Source: CAD feature listing. Evaluate the final solid. Frame: model axes, mm. A direction names the side the tool comes from. Give positions to 0.01 mm unless a question says otherwise; leave off trailing zeros. Order: outer loops, then holes, each group sorted by start corner. A loop starts at its lowest first (then second) coordinate and runs counter-clockwise, first axis right, second up.
1) Section C-C, the plane z = -31. Return loops of the section in (x, y).
2) Draft query along X for faces 3 (the face through (-50.503, 3.042, -109.333)), 4 (the face through (-2, 3, 138)). Return one class per face: released by +X, released by -X, zero draft, split by the parting line, or undercut.
3) Material intervals for line 1 (X direction, y = 2.4, z = 55); line 2 (Z direction, x = 128, y = 4.35); line 3 (X direction, y = 2.6, z = -60), sorted ascending.
4) Section A-A, the plane x = -66.5. Return loops of the section in (y, z), plus the area to 3 significant figures.
5) Section B-B, the plane z = 35.5. Return loops of the section in (x, y), plus the area to 3 significant figures.
6) Access query for faces 1 (the face through (2.377, 3.042, -33.695)), 2 (the face through (-2, 3, -138)). Directions: +Z, -Z, +X, -X, +Y, -Y. A direction counts if a zero-diameter tool reaches every point of the face in a straight line with its end or side. Return the directions, or none.
7) Section D-D, the plane y = 1.35. Give the number of separate pieces and of enclosed holes in the cut face, plus the area to 3 significant figures.
```python
from build123d import *

# Parameters (mm, degrees)
SKETCH_1_W                = 276
SKETCH_1_H                = 276
EXTRUDE_1_DEPTH           = 6
FILLET_1_R                = 2
SKETCH_2_R                = 2
CUT_EXTRUDE_1_DEPTH       = 6
SKETCH_3_R                = 2
CUT_EXTRUDE_150_164_DEPTH = 6
SKETCH_4_R                = 2
CUT_EXTRUDE_94_94_DEPTH   = 6
SKETCH_7_R                = 1.75
JETSON_DEPTH              = 6
SKETCH_8_R                = 1.75
CUT_EXTRUDE_7_DEPTH       = 6
SKETCH_9_R                = 1.8
CUT_EXTRUDE_8_DEPTH       = 6
CUT_EXTRUDE_5_DEPTH       = 6


with BuildPart() as part:
    # Эскиз1 → Бобышка-Вытянуть1 (new body)
    with BuildSketch(Plane(origin=(0, 0, 0), x_dir=(1, 0, 0), z_dir=(0, 1, 0))):
        Rectangle(SKETCH_1_W, SKETCH_1_H)
    extrude(amount=EXTRUDE_1_DEPTH)

    # Скругление1
    fillet_1_edges = [part.edges().sort_by_distance(p)[0] for p in [
        (138, 3, 138),
        (-138, 3, 138),
        (-138, 3, -138),
        (138, 3, -138),
    ]]
    fillet(fillet_1_edges, radius=FILLET_1_R)

    # Эскиз2 → Вырез-Вытянуть1 (cut)
    with BuildSketch(Plane(origin=(0, 6, 0), x_dir=(1, 0, 0), z_dir=(0, 1, 0))):
        with Locations(Location((-134, 60, 0), (0, 0, 270))):
            Circle(SKETCH_2_R)
        with Locations(Location((134, 60, 0), (0, 0, 90))):
            Circle(SKETCH_2_R)
        with Locations(Location((134, -60, 0), (0, 0, 270))):
            Circle(SKETCH_2_R)
        with Locations(Location((-134, -60, 0), (0, 0, 90))):
            Circle(SKETCH_2_R)
        with Locations(Location((46, 60, 0), (0, 0, 270))):
            Circle(SKETCH_2_R)
        with Locations(Location((46, -60, 0), (0, 0, 90))):
            Circle(SKETCH_2_R)
        with Locations(Location((134, 134, 0), (0, 0, 270))):
            Circle(SKETCH_2_R)
        with Locations(Location((134, -134, 0), (0, 0, 90))):
            Circle(SKETCH_2_R)
    extrude(amount=-CUT_EXTRUDE_1_DEPTH, mode=Mode.SUBTRACT)

    # Эскиз3 → 150х164 (cut)
    with BuildSketch(Plane(origin=(0, 6, 0), x_dir=(1, 0, 0), z_dir=(0, 1, 0))):
        with Locations(Location((-32, 82, 0), (0, 0, 270))):
            Circle(SKETCH_3_R)
        with Locations(Location((118, 82, 0), (0, 0, 270))):
            Circle(SKETCH_3_R)
        with Locations(Location((125, 75, 0), (0, 0, 270))):
            Circle(SKETCH_3_R)
        with Locations(Location((-39, 75, 0), (0, 0, 270))):
            Circle(SKETCH_3_R)
        with Locations(Location((118, -82, 0), (0, 0, 90))):
            Circle(SKETCH_3_R)
        with Locations(Location((125, -75, 0), (0, 0, 90))):
            Circle(SKETCH_3_R)
        with Locations(Location((-32, -82, 0), (0, 0, 90))):
            Circle(SKETCH_3_R)
        with Locations(Location((-39, -75, 0), (0, 0, 90))):
            Circle(SKETCH_3_R)
        with Locations(Location((-124, 75, 0), (0, 0, 270))):
            Circle(SKETCH_3_R)
        with Locations(Location((40, 75, 0), (0, 0, 270))):
            Circle(SKETCH_3_R)
        with Locations(Location((33, 82, 0), (0, 0, 270))):
            Circle(SKETCH_3_R)
        with Locations(Location((40, -75, 0), (0, 0, 270))):
            Circle(SKETCH_3_R)
        with Locations(Location((33, -82, 0), (0, 0, 270))):
            Circle(SKETCH_3_R)
        with Locations(Location((-117, -82, 0), (0, 0, 270))):
            Circle(SKETCH_3_R)
        with Locations(Location((-124, -75, 0), (0, 0, 270))):
            Circle(SKETCH_3_R)
        with Locations(Location((-117, 82, 0), (0, 0, 90))):
            Circle(SKETCH_3_R)
    extrude(amount=-CUT_EXTRUDE_150_164_DEPTH, mode=Mode.SUBTRACT)

    # Эскиз4 → 94х94 (cut)
    with BuildSketch(Plane(origin=(0, 6, 0), x_dir=(1, 0, 0), z_dir=(0, 1, 0))):
        with Locations(Location((-128, 107, 0), (0, 0, 270))):
            Circle(SKETCH_4_R)
        with Locations(Location((-34, 107, 0), (0, 0, 270))):
            Circle(SKETCH_4_R)
        with Locations(Location((-34, 13, 0), (0, 0, 90))):
            Circle(SKETCH_4_R)
        with Locations(Location((-128, 13, 0), (0, 0, 90))):
            Circle(SKETCH_4_R)
        with Locations(Location((-128, -13, 0), (0, 0, 270))):
            Circle(SKETCH_4_R)
        with Locations(Location((-34, -13, 0), (0, 0, 270))):
            Circle(SKETCH_4_R)
        with Locations(Location((-34, -107, 0), (0, 0, 90))):
            Circle(SKETCH_4_R)
        with Locations(Location((-128, -107, 0), (0, 0, 90))):
            Circle(SKETCH_4_R)
    extrude(amount=-CUT_EXTRUDE_94_94_DEPTH, mode=Mode.SUBTRACT)

    # Эскиз7 → Jetson (cut)
    with BuildSketch(Plane(origin=(0, 6, 0), x_dir=(1, 0, 0), z_dir=(0, 1, 0))):
        with Locations(Location((-18, 78, 0), (0, 0, 270))):
            Circle(SKETCH_7_R)
        with Locations(Location((-18, 26, 0), (0, 0, 270))):
            Circle(SKETCH_7_R)
        with Locations(Location((98, 78, 0), (0, 0, 270))):
            Circle(SKETCH_7_R)
        with Locations(Location((98, 26, 0), (0, 0, 270))):
            Circle(SKETCH_7_R)
    extrude(amount=-JETSON_DEPTH, mode=Mode.SUBTRACT)

    # Эскиз8 → Вырез-Вытянуть7 (cut)
    with BuildSketch(Plane(origin=(0, 6, 0), x_dir=(1, 0, 0), z_dir=(0, 1, 0))):
        with Locations(Location((48, -79, 0), (0, 0, 270))):
            Circle(SKETCH_8_R)
        with Locations(Location((-10, -79, 0), (0, 0, 270))):
            Circle(SKETCH_8_R)
        with Locations(Location((-10, -128, 0), (0, 0, 270))):
            Circle(SKETCH_8_R)
        with Locations(Location((48, -128, 0), (0, 0, 270))):
            Circle(SKETCH_8_R)
    extrude(amount=-CUT_EXTRUDE_7_DEPTH, mode=Mode.SUBTRACT)

    # Эскиз9 → Вырез-Вытянуть8 (cut)
    with BuildSketch(Plane(origin=(0, 6, 0), x_dir=(1, 0, 0), z_dir=(0, 1, 0))):
        with Locations(Location((-7, 2, 0), (0, 0, 270))):
            Circle(SKETCH_9_R)
        with Locations(Location((43, 2, 0), (0, 0, 270))):
            Circle(SKETCH_9_R)
        with Locations(Location((83, 2, 0), (0, 0, 270))):
            Circle(SKETCH_9_R)
        with Locations(Location((123, 2, 0), (0, 0, 270))):
            Circle(SKETCH_9_R)
        with Locations(Location((123, -48, 0), (0, 0, 90))):
            Circle(SKETCH_9_R)
        with Locations(Location((83, -48, 0), (0, 0, 90))):
            Circle(SKETCH_9_R)
        with Locations(Location((43, -48, 0), (0, 0, 90))):
            Circle(SKETCH_9_R)
        with Locations(Location((-7, -48, 0), (0, 0, 90))):
            Circle(SKETCH_9_R)
        with Locations(Location((43, -23, 0), (0, 0, 270))):
            Circle(SKETCH_9_R)
        with Locations(Location((-7, -23, 0), (0, 0, 270))):
            Circle(SKETCH_9_R)
        with Locations(Location((83, -23, 0), (0, 0, 270))):
            Circle(SKETCH_9_R)
        with Locations(Location((123, -23, 0), (0, 0, 270))):
            Circle(SKETCH_9_R)
        with Locations(Location((123, 62, 0), (0, 0, 270))):
            Circle(SKETCH_9_R)
        with Locations(Location((123, 122, 0), (0, 0, 270))):
            Circle(SKETCH_9_R)
        with Locations(Location((123, -108, 0), (0, 0, 90))):
            Circle(SKETCH_9_R)
        with Locations(Location((98, 13, 0), (0, 0, 270))):
            Circle(SKETCH_9_R)
        with Locations(Location((128, 13, 0), (0, 0, 270))):
            Circle(SKETCH_9_R)
        with Locations(Location((98, -17, 0), (0, 0, 270))):
            Circle(SKETCH_9_R)
        with Locations(Location((128, -17, 0), (0, 0, 270))):
            Circle(SKETCH_9_R)
        with Locations(Location((98, -29, 0), (0, 0, 90))):
            Circle(SKETCH_9_R)
        with Locations(Location((128, -29, 0), (0, 0, 90))):
            Circle(SKETCH_9_R)
        with Locations(Location((128, -59, 0), (0, 0, 90))):
            Circle(SKETCH_9_R)
        with Locations(Location((98, -59, 0), (0, 0, 90))):
            Circle(SKETCH_9_R)
    extrude(amount=-CUT_EXTRUDE_8_DEPTH, mode=Mode.SUBTRACT)

    # Эскиз6 → Вырез-Вытянуть5 (cut)
    with BuildSketch(Plane(origin=(0, 6, 0), x_dir=(1, 0, 0), z_dir=(0, 1, 0))):
        with BuildLine():
            Line((-103, 97.107947115), (-63, 97.107947115))
            ThreePointArc((-63, 97.107947115), (-50.5, 109.607947115), (-63, 122.107947115))
            Line((-63, 122.107947115), (-103, 122.107947115))
            ThreePointArc((-103, 122.107947115), (-115.5, 109.607947115), (-103, 97.107947115))
        make_face()
        with BuildLine():
            ThreePointArc((-70.5, 23), (-83, 10.5), (-95.5, 23))
            Line((-95.5, 23), (-95.5, 73))
            ThreePointArc((-95.5, 73), (-83, 85.5), (-70.5, 73))
            Line((-70.5, 73), (-70.5, 23))
        make_face()
        with BuildLine():
            Line((-70.5, -73), (-70.5, -23))
            ThreePointArc((-70.5, -23), (-83, -10.5), (-95.5, -23))
            Line((-95.5, -23), (-95.5, -73))
            ThreePointArc((-95.5, -73), (-83, -85.5), (-70.5, -73))
        make_face()
        with BuildLine():
            ThreePointArc((-63, -97.107947115), (-50.5, -109.607947115), (-63, -122.107947115))
            Line((-63, -122.107947115), (-103, -122.107947115))
            ThreePointArc((-103, -122.107947115), (-115.5, -109.607947115), (-103, -97.107947115))
            Line((-103, -97.107947115), (-63, -97.107947115))
        make_face()
        with BuildLine():
            Line((16.282052685, 19.480778886), (69.672016653, 19.480778886))
            ThreePointArc((69.672016653, 19.480778886), (83.580326595, 33.389088828), (69.672016653, 47.297398769))
            Line((69.672016653, 47.297398769), (16.282052685, 47.297398769))
            ThreePointArc((16.282052685, 47.297398769), (2.373742744, 33.389088828), (16.282052685, 19.480778886))
        make_face()
        with BuildLine():
            Line((73.817325583, -73.648631168), (73.817325583, -114.962929045))
            ThreePointArc((73.817325583, -114.962929045), (83.686480688, -124.832084149), (93.555635792, -114.962929045))
            Line((93.555635792, -114.962929045), (93.555635792, -73.648631168))
            ThreePointArc((93.555635792, -73.648631168), (83.686480688, -63.779476064), (73.817325583, -73.648631168))
        make_face()
        with BuildLine():
            ThreePointArc((20, -97.107947115), (32.5, -109.607947115), (20, -122.107947115))
            Line((20, -122.107947115), (-10, -122.107947115))
            ThreePointArc((-10, -122.107947115), (-22.5, -109.607947115), (-10, -97.107947115))
            Line((-10, -97.107947115), (20, -97.107947115))
        make_face()
        with BuildLine():
            Line((-10, 97.107947115), (20, 97.107947115))
            ThreePointArc((20, 97.107947115), (32.5, 109.607947115), (20, 122.107947115))
            Line((20, 122.107947115), (-10, 122.107947115))
            ThreePointArc((-10, 122.107947115), (-22.5, 109.607947115), (-10, 97.107947115))
        make_face()
    extrude(amount=-CUT_EXTRUDE_5_DEPTH, mode=Mode.SUBTRACT)


solid = part.part
```
From the geometry:
1. outline: (-138, 0) - (-95.5, 0) - (-95.5, 6) - (-138, 6) - close; (-70.5, 0) - (2.58, 0) - (2.58, 6) - (-70.5, 6) - close; (83.37, 0) - (138, 0) - (138, 6) - (83.37, 6) - close
2. face 3: undercut
2. face 4: zero draft
3. line 1: x = -138 to -95.5, -70.5 to 138
3. line 2: z = -138 to -14.8, -11.2 to 15.2, 18.8 to 27.2, 30.8 to 57.2, 60.8 to 138
3. line 3: x = -138 to -136, -132 to -95.5, -70.5 to 44, 48 to 132, 136 to 138
4. outline: (0, -138) - (6, -138) - (6, -122.11) - (0, -122.11) - close; (0, -97.11) - (6, -97.11) - (6, 97.11) - (0, 97.11) - close; (0, 122.11) - (6, 122.11) - (6, 138) - (0, 138) - close
4. area: 1,360 mm2
5. outline: (-138, 0) - (-95.5, 0) - (-95.5, 6) - (-138, 6) - close; (-70.5, 0) - (138, 0) - (138, 6) - (-70.5, 6) - close
5. area: 1,510 mm2
6. face 1: +Y, -Y
6. face 2: -Z, +X, -X, +Y, -Y
7. separate pieces: 1
7. enclosed holes: 71
7. area: 63,300 mm2
